from build123d import *

# Parameters (mm, degrees)
SKETCH_1_R          = 3
EXTRUDE_1_DEPTH     = 5
EXTRUDE_2_DEPTH     = 2.5
EXTRUDE_3_DEPTH     = 5.5
EXTRUDE_3_TAPER     = 27
SKETCH_5_R          = 0.05
CUT_EXTRUDE_1_DEPTH = 14.792224458
SKETCH_6_R          = 2.127494577
CUT_EXTRUDE_2_DEPTH = 7.5
CUT_EXTRUDE_2_DRAFT = -15


with BuildPart() as part:
    # 草图1 → 凸台-拉伸1 (new body)
    with BuildSketch(Plane(origin=(0, 0, 0), x_dir=(1, 0, 0), z_dir=(0, 1, 0))):
        with Locations(Location((0, 0, 0), (0, 0, 270))):
            Circle(SKETCH_1_R)
    extrude(amount=EXTRUDE_1_DEPTH)

    # 草图2 → 凸台-拉伸2 (add)
    with BuildSketch(Plane(origin=(0, 5, 0), x_dir=(1, 0, 0), z_dir=(0, 1, 0))):
        Polygon((3.038350598, -1.663858661), (2.960119168, 1.799359473), (-0.07823143, 3.463218134), (-3.038350598, 1.663858661), (-2.960119168, -1.799359473), (0.07823143, -3.463218134), align=None)
    extrude(amount=EXTRUDE_2_DEPTH)

    # 草图4 → 凸台-拉伸3 (add)
    with BuildSketch(Plane(origin=(0, 7.5, 0), x_dir=(1, 0, 0), z_dir=(0, 1, 0))):
        Polygon((0.07823143, -3.463218134), (3.038350598, -1.663858661), (2.960119168, 1.799359473), (-0.07823143, 3.463218134), (-3.038350598, 1.663858661), (-2.960119168, -1.799359473), align=None)
    extrude(amount=EXTRUDE_3_DEPTH, taper=EXTRUDE_3_TAPER)

    # 草图5 → 切除-拉伸1 (cut, through all)
    with BuildSketch(Plane(origin=(0, 13, 0), x_dir=(1, 0, 0), z_dir=(0, 1, 0))):
        with Locations(Location((0, 0, 0), (0, 0, 270))):
            Circle(SKETCH_5_R)
    extrude(amount=-CUT_EXTRUDE_1_DEPTH, mode=Mode.SUBTRACT)


with BuildPart() as cut_extrude_2_tool:
    # 草图6 → 切除-拉伸2 (with draft: the straight prism first)
    with BuildSketch(Plane.XZ):
        with Locations((-0.05, 0)):
            Circle(SKETCH_6_R)
    extrude(amount=-CUT_EXTRUDE_2_DEPTH)
    # 切除-拉伸2: the draft: its side faces are tilted about the plane it starts from
    cut_extrude_2_sides = [cut_extrude_2_tool.faces().sort_by_distance(p)[0] for p in [
        (-2.177494577, 3.75, 0),
    ]]
    draft(cut_extrude_2_sides, Plane.XZ, CUT_EXTRUDE_2_DRAFT)


with BuildPart() as part_1:
    add(part.part)

    # 切除-拉伸2: cut by cut_extrude_2_tool
    add(cut_extrude_2_tool.part, mode=Mode.SUBTRACT)


solid = part_1.part
Geometry check sheet. Reference: the model listing, model coordinates, mm. A direction names the side the tool comes from. Coordinates: 2 decimals unless noted, no trailing zeros. Write each loop counter-clockwise with the first axis right and the second up, starting at its lowest first coordinate (ties: lowest second). Pieces come first, ordered by that corner, then holes. Notation, with made-up numbers: (-33, -12.5) -> (-1, -12.5) arc R20 cw to (-1, 3.5) -> close; hole circle Ø1 at (81, 30). An arc over 180 degrees is marked (long way). One line per question, with ' | ' between items.
1. Depth check by flat-ended pin: pin 1 Ø3 at (x, y) = (-1, 11.5) entering from +Z; pin 2 Ø1 at (y, z) = (5, 0) entering from -X; pin 3 Ø1.5 at (x, y) = (2, 5.5) entering from -Z. Enter the tip coordinate at first touch or a pass-through.
Answers:
pin 1: stops at z = 1.75 | pin 2: stops at x = -3.01 | pin 3: stops at z = -2.74
2. Thickness scan on probe 1 along Y at (x, z) = (-2.25, 1); probe 2 along Y at (x, z) = (-2, -1); probe 3 along X at (y, z) = (8.75, 2.5). Record the ranges inside material, lowest first. Write a range as from..to.
Answers:
probe 1: y = 0..8.93 | probe 2: y = 0..9.51 | probe 3: x = -0.35..0.44
3. Draft check along X on faces 1 (the cylindrical face through (0.9, 2.46, 2.86)), 2 (the flat face through (2.74, 5, -1.64)), 3 (the conical face through (1.034, 3.698, 0.341)). Enter one of: +X half, -X half, draft (parallel to the pull), parting line (faces both ways), or undercut.
Answers:
face 1: parting line | face 2: draft | face 3: undercut
4. Cross-section at A-A on y = 7. Record the cut outline in (x, z), and give its area (3 significant figures).
Answers:
outline: (-3.04, -1.66) -> (-0.08, -3.46) -> (2.96, -1.8) -> (3.04, 1.66) -> (0.08, 3.46) -> (-2.96, 1.8) -> close; hole circle Ø0.5 at (-0.05, 0) | area: 31.0 mm²
5. Set-up check for faces 4 (the flat face through (-2.74, 5, 1.63)), 5 (the flat face through (-2.8, 5, -1.5)), 6 (the flat face through (2.8, 5, 1.5)): record each of +Z, -Z, +X, -X, +Y, -Y from which the full face is reachable in a straight line by a thin tool's end or side.
Answers:
face 4: +Z, -X, -Y | face 5: -Z, -X, -Y | face 6: +Z, +X, -Y
6. Cross-section at C-C on y = 3. Record the cut outline in (x, z), and give its area (3 significant figures).
Answers:
outline: circle Ø6 at (0, 0); hole circle Ø2.65 at (-0.05, 0) | area: 22.8 mm²
7. Cross-section at B-B on y = 4.5. Record the cut outline in (x, z).
Answers:
outline: circle Ø6 at (0, 0); hole circle Ø1.84 at (-0.05, 0)
